from build123d import *

# Parameters (mm, degrees)
F0_W     = 19.05
F0_H     = 19.05
F1_DEPTH = 25.4
F2_W     = 19.05
F2_H     = 19.05
F3_DEPTH = 6.35
F4_R     = 0.889
F5_DEPTH = 19.05


with BuildPart() as f1:
    # F0 (on Front) → F1 (new body)
    with BuildSketch(Plane.XZ):
        Polygon((12.7, -12.7), (12.7, 12.7), (11.176, 12.7), (-11.176, 12.7), (-12.7, 12.7), (-12.7, -12.7), (-11.176, -12.7), (11.176, -12.7), align=None)
        with BuildLine():
            ThreePointArc((-10.284095511, -11.1804986587), (-10.5455053146, -11.8101426417), (-11.176, -12.069493914))
            ThreePointArc((-11.176, -12.069493914), (-11.8006857075, -10.5508546757), (-10.284095511, -11.1804986587))
        make_face(mode=Mode.SUBTRACT)
        Rectangle(F0_W, F0_H, mode=Mode.SUBTRACT)
        with BuildLine():
            ThreePointArc((12.0763947175, -11.1804986587), (11.8119710123, -11.813132401), (11.176, -12.0694256301))
            ThreePointArc((11.176, -12.0694256301), (10.5628184227, -10.5478649164), (12.0763947175, -11.1804986587))
        make_face(mode=Mode.SUBTRACT)
        with BuildLine():
            ThreePointArc((-10.2897327763, 11.1719880705), (-11.8083161457, 10.5443370679), (-11.176, 12.0609838702))
            ThreePointArc((-11.176, 12.0609838702), (-10.5491494068, 11.799639073), (-10.2897327763, 11.1719880705))
        make_face(mode=Mode.SUBTRACT)
        with BuildLine():
            ThreePointArc((12.065, 11.176), (10.5473820715, 10.5473820715), (11.176, 12.065))
            ThreePointArc((11.176, 12.065), (11.8046179285, 11.8046179285), (12.065, 11.176))
        make_face(mode=Mode.SUBTRACT)
    extrude(amount=F1_DEPTH)

    # F2 (on Front) → F3 (join)
    with BuildSketch(Plane.XZ):
        Rectangle(F2_W, F2_H)
    extrude(amount=F3_DEPTH)

    # F4 (on face) → F5 (join)
    with BuildSketch(Plane(origin=(0, 0, 0), x_dir=(-1, 0, 0), z_dir=(0, 1, 0))):
        with Locations((11.1787327763, 11.1719880705)):
            Circle(F4_R)
        with Locations((-11.1873947175, -11.1804986587)):
            Circle(F4_R)
        with Locations((11.173095511, -11.1804986587)):
            Circle(F4_R)
        with Locations((-11.176, 11.176)):
            Circle(F4_R)
    extrude(amount=-F5_DEPTH)


solid = f1.part
The listing builds one solid part. Answer for the finished solid, in the listing's coordinates (mm). A direction names the side the tool comes from. Give positions to 0.01 mm unless a question says otherwise; leave off trailing zeros. Loops run counter-clockwise (first coordinate to the right, second up) from the corner with the lowest first, then second, coordinate; pieces in that order, holes last. Notation, with made-up numbers: (-20.5, 50) - (-3.5, 50) arc R26 ccw to (-3.5, 72) - close; hole circle Ø4 at (35, 66). An arc over 180 degrees is marked (long way). Use one line per item in the form item = value.
1. Section A-A on z = 0.25 is taken. Give the vertices of the cut face in (x, y) (3 decimals).
Calculated:
outline = (-12.7, -25.4) - (-9.525, -25.4) - (-9.525, -6.35) - (9.525, -6.35) - (9.525, -25.4) - (12.7, -25.4) - (12.7, 0) - (-12.7, 0) - close
2. Section B-B on y = -22 is taken. Give the vertices of the cut face in (x, z) (1 decimal).
Calculated:
outline = (-12.7, -12.7) - (12.7, -12.7) - (12.7, 12.7) - (-12.7, 12.7) - close; hole circle Ø1.8 at (-11.2, -11.2); hole circle Ø1.8 at (-11.2, 11.2); hole (-9.5, -9.5) - (9.5, -9.5) - (9.5, 9.5) - (-9.5, 9.5) - close; hole circle Ø1.8 at (11.2, -11.2); hole circle Ø1.8 at (11.2, 11.2)
3. Which of the six approach directions +Z, -Z, +X, -X, +Y, -Y give full straight-line access (tool end or side, diameter ignored) to faces 1 (the face through (-11, -19.05, 11)), 2 (the face through (0, -13, -12.7))?
Calculated:
face_1 = -Y
face_2 = -Z, +X, -X, +Y, -Y
4. Given pin 1 Ø0.5 at (x, z) = (-11, -11.5) entering from -Y; pin 2 Ø2 at (x, z) = (0, 5.5) entering from -Y, each flat-ended and moving along its own axis, determine where each tip first touches the part or whether it passes through.
Calculated:
pin_1 = -19.05
pin_2 = -6.35
5. Find the intervals of material crossed by line 1 along Z through (x, y) = (-0.75, -18.5) (3 decimals); line 2 along Y through (x, z) = (1.75, -3), in increasing order. Write a range as [from, to].
Calculated:
line_1 = [-12.7, -9.525], [9.525, 12.7]
line_2 = [-6.35, 0]
6. Section C-C on y = -18.5 is taken. Give the vertices of the cut face in (x, z) (3 decimals).
Calculated:
outline = (-12.7, -12.7) - (12.7, -12.7) - (12.7, 12.7) - (-12.7, 12.7) - close; hole (-9.525, -9.525) - (9.525, -9.525) - (9.525, 9.525) - (-9.525, 9.525) - close
7. The mould has two halves that part along X. Classify faces 3 (the face through (-12.7, -13, 0)), 4 (the face through (9.525, -16, 0)), 5 (the face through (0, -13, 12.7)), 6 (the face through (0, -16, 9.525)): pulls with the +X half, pulls with the -X half, needs draft (parallel to the pull), parting line crosses it, or undercut.
Calculated:
face_3 = pulls with the -X half
face_4 = undercut
face_5 = needs draft
face_6 = undercut
8. Section D-D on x = -8 is taken. Give the vertices of the cut face in (y, z) (3 decimals), then the cut area to 3 significant figures.
Calculated:
outline = (-25.4, -12.7) - (0, -12.7) - (0, 12.7) - (-25.4, 12.7) - (-25.4, 9.525) - (-6.35, 9.525) - (-6.35, -9.525) - (-25.4, -9.525) - close
area = 282 mm^2
